```python
from build123d import *

# Parameters (mm, degrees)
SKETCH1_W                = 7.4
SKETCH1_H                = 5.75
BOSS_EXTRUDE1_DEPTH      = 7
SHELL1_T                 = -0.8
SKETCH2_W                = 1.25
SKETCH2_H                = 3.2
CUT_EXTRUDE1_DEPTH       = 8.4
CUT_EXTRUDE2_REACH       = 7.75
SKETCH3_W                = 3.6
SKETCH3_H                = 3.8
SKETCH4_W                = 0.64
SKETCH4_H                = 0.64
BOSS_EXTRUDE2_DEPTH      = 3.45
BOSS_EXTRUDE2_DEPTH_BACK = 6.75
CHAMFER1_SIZE            = 0.2


with BuildPart() as part:
    # Sketch1 → Boss-Extrude1 (new body)
    with BuildSketch(Plane(origin=(0, 0, 0), x_dir=(1, 0, 0), z_dir=(0, 1, 0))):
        Rectangle(SKETCH1_W, SKETCH1_H)
    extrude(amount=BOSS_EXTRUDE1_DEPTH)

    # Shell1
    shell1_openings = [part.faces().sort_by_distance(p)[0] for p in [
        (0, 7, 0),
    ]]
    offset(amount=SHELL1_T, openings=shell1_openings, kind=Kind.INTERSECTION)

    # Sketch2 → Cut-Extrude1 (cut, through all)
    with BuildSketch(Plane(origin=(3.7, 0, 0), x_dir=(0, 0, -1), z_dir=(1, 0, 0))):
        with Locations((-1.5, 5.4)):
            Rectangle(SKETCH2_W, SKETCH2_H)
    extrude(amount=-CUT_EXTRUDE1_DEPTH, mode=Mode.SUBTRACT)

    # Sketch3 → Cut-Extrude2 (cut, up to next)
    with BuildSketch(Plane.XY.offset(2.875), mode=Mode.PRIVATE) as cut_extrude2_sk1:
        with Locations((0, 5.1)):
            Rectangle(SKETCH3_W, SKETCH3_H)
    cut_extrude2_tool1 = extrude(cut_extrude2_sk1.sketch, amount=-CUT_EXTRUDE2_REACH, mode=Mode.PRIVATE) & part.part
    add(cut_extrude2_tool1.solids().sort_by_distance((0, 5.1, 2.875))[0], mode=Mode.SUBTRACT)

    # Sketch4 → Boss-Extrude2 (add, two sides)
    with BuildSketch(Plane.XZ) as boss_extrude2_sk:
        with Locations((-1.25, 0.525)):
            Rectangle(SKETCH4_W, SKETCH4_H)
        with Locations((1.25, 0.525)):
            Rectangle(SKETCH4_W, SKETCH4_H)
    extrude(amount=BOSS_EXTRUDE2_DEPTH)
    extrude(boss_extrude2_sk.sketch, amount=-BOSS_EXTRUDE2_DEPTH_BACK)

    # Chamfer1
    chamfer1_edges = [part.edges().sort_by_distance(p)[0] for p in [
        (-0.93, 6.75, 0.525),
        (-1.25, 6.75, 0.205),
        (-1.57, 6.75, 0.525),
        (-1.25, 6.75, 0.845),
        (-0.93, -3.45, 0.525),
        (-1.25, -3.45, 0.845),
        (-1.57, -3.45, 0.525),
        (-1.25, -3.45, 0.205),
        (1.25, 6.75, 0.845),
        (1.57, 6.75, 0.525),
        (1.25, 6.75, 0.205),
        (0.93, 6.75, 0.525),
        (1.25, -3.45, 0.845),
        (0.93, -3.45, 0.525),
        (1.25, -3.45, 0.205),
        (1.57, -3.45, 0.525),
    ]]
    chamfer(chamfer1_edges, length=CHAMFER1_SIZE)


solid = part.part
```
Input: part model. Units: mm. Frame: model coordinates. A direction names the side the tool comes from. Give positions to 0.01 mm unless a question says otherwise; leave off trailing zeros. Loops run counter-clockwise (first coordinate to the right, second up) from the corner with the lowest first, then second, coordinate; pieces in that order, holes last. Notation, with made-up numbers: (47, 0.5) -> (101, 0.5) arc R29 ccw to (101, 24.5) -> close; hole circle Ø10 at (28, 30.5). An arc over 180 degrees is marked (long way). Use a Markdown table: item, result.
Q1. Pull-direction query (X, two-part tool) for faces 4 (the flat face through (0, 0.8, 0)), 5 (the flat face through (-3.2, 3.8, 1.5)), 6 (the flat face through (2.9, 4, 0)), 7 (the flat face through (3.7, 3, 0)); classes: pulls with the +X half, pulls with the -X half, needs draft (parallel to the pull), parting line crosses it, or undercut.
Entries:
| item | result |
|---|---|
| face 4 | undercut |
| face 5 | needs draft |
| face 6 | undercut |
| face 7 | pulls with the +X half |
Q2. Ray query, probe 1 along X at (y, z) = (2, 0.7); probe 2 along Z at (x, y) = (2, 1.5) (3 decimals); probe 3 along Z at (x, y) = (1.25, 1.25) (3 decimals). Return the intervals inside material, ascending. Write a range as from..to.
Entries:
| item | result |
|---|---|
| probe 1 | x = -3.7..-2.9, -1.57..-0.93, 0.93..1.57, 2.9..3.7 |
| probe 2 | z = -2.875..-2.075, 2.075..2.875 |
| probe 3 | z = -2.875..-2.075, 0.205..0.845, 2.075..2.875 |
Q3. Section query A-A, the plane y = 3. Return the cut outline in (x, z) (3 decimals).
Entries:
| item | result |
|---|---|
| outline | (-3.7, -2.875) -> (3.7, -2.875) -> (3.7, 2.875) -> (-3.7, 2.875) -> close; (-1.57, 0.205) -> (-0.93, 0.205) -> (-0.93, 0.845) -> (-1.57, 0.845) -> close; (0.93, 0.205) -> (1.57, 0.205) -> (1.57, 0.845) -> (0.93, 0.845) -> close; hole (-2.9, -2.075) -> (2.9, -2.075) -> (2.9, 2.075) -> (-2.9, 2.075) -> close |
Q4. Section query D-D, the plane z = -0.4. Return the cut outline in (x, y), plus the area to 3 significant figures.
Entries:
| item | result |
|---|---|
| outline | (-3.7, 0) -> (3.7, 0) -> (3.7, 7) -> (2.9, 7) -> (2.9, 0.8) -> (-2.9, 0.8) -> (-2.9, 7) -> (-3.7, 7) -> close |
| area | 15.8 mm² |
Q5. Access query for faces 1 (the flat face through (0, 3, 2.875)), 2 (the flat face through (-2.9, 4, 0)), 3 (the flat face through (-3, 5, 2.125)). Directions: +Z, -Z, +X, -X, +Y, -Y. A direction counts if a zero-diameter tool reaches every point of the face in a straight line with its end or side. Return the directions, or none.
Entries:
| item | result |
|---|---|
| face 1 | +Z, +X, -X, +Y, -Y |
| face 2 | +Y |
| face 3 | +X, -X, +Y |
Q6. Section query C-C, the plane x = 0.5. Return the cut outline in (y, z) (3 decimals).
Entries:
| item | result |
|---|---|
| outline | (0, -2.875) -> (7, -2.875) -> (7, -2.075) -> (0.8, -2.075) -> (0.8, 2.075) -> (3.2, 2.075) -> (3.2, 2.875) -> (0, 2.875) -> close |
Q7. First-contact query: P1, Ø0.7, axis at y = -1, z = 0.5, coming from the -X side; P2, Ø0.5, axis at x = 1.5, y = -1, coming from the +Z side (3 decimals); P3, Ø2, axis at x = -2.5, z = 0, coming from the -Y side. Flat tips, straight axial feed; report the tip coordinate or a pass-through.
Entries:
| item | result |
|---|---|
| P1 | stops at x = -1.57 |
| P2 | stops at z = 0.845 |
| P3 | stops at y = -3.29 |
Q8. Section query B-B, the plane y = -1.5. Return the cut outline in (x, z) (3 decimals).
Entries:
| item | result |
|---|---|
| outline | (-1.57, 0.205) -> (-0.93, 0.205) -> (-0.93, 0.845) -> (-1.57, 0.845) -> close; (0.93, 0.205) -> (1.57, 0.205) -> (1.57, 0.845) -> (0.93, 0.845) -> close |
